For this review, use the dimensioned drawing (mm, ordinates from the lowest corner) and the shaded views. Round coordinates to 2 decimals unless told otherwise and drop trailing zeros. Write each loop counter-clockwise with the first axis right and the second up, starting at its lowest first coordinate (ties: lowest second). Pieces come first, ordered by that corner, then holes. Notation, with made-up numbers: (-28, 20) - (23, 20) arc R6 ccw to (23, 31) - close; hole circle Ø1 at (27, 44.25). An arc over 180 degrees is marked (long way). Write each question's results on one line, items separated by ' | '.
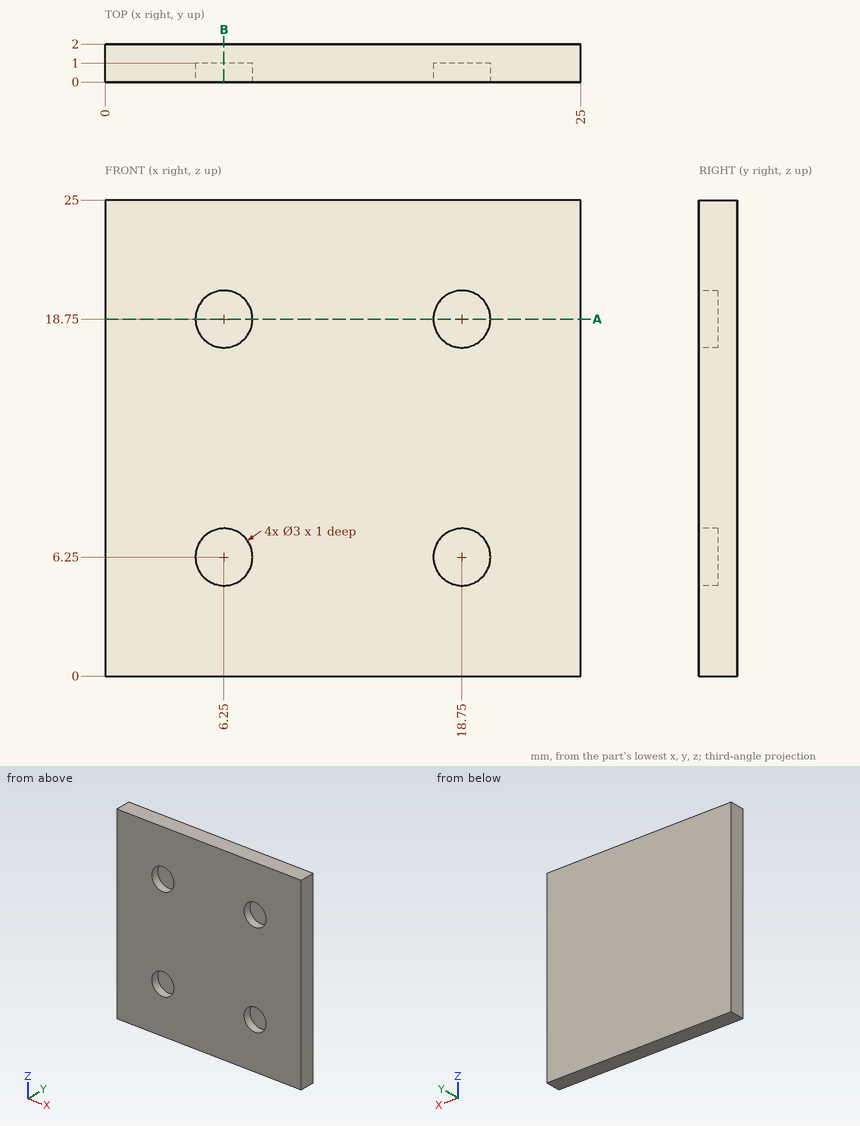
Q1. For probe 1 along Z at (x, y) = (18.75, 0.6); probe 2 along X at (y, z) = (0.75, 7); probe 3 along Z at (x, y) = (7.5, 0.1), list the stretches that pass through material, from the lowest coordinate up.
Evaluation:
probe 1: z = 0 to 4.75, 7.75 to 17.25, 20.25 to 25 | probe 2: x = 0 to 4.95, 7.55 to 17.45, 20.05 to 25 | probe 3: z = 0 to 5.42, 7.08 to 17.92, 19.58 to 25
Q2. We need section A-A (z = 18.75). State the section outline as (x, y) points.
Evaluation:
outline: (0, 0) - (4.75, 0) - (4.75, 1) - (7.75, 1) - (7.75, 0) - (17.25, 0) - (17.25, 1) - (20.25, 1) - (20.25, 0) - (25, 0) - (25, 2) - (0, 2) - close
Q3. We need section B-B (x = 6.25). State the section outline as (y, z) points, plus the area to 3 significant figures.
Evaluation:
outline: (0, 0) - (2, 0) - (2, 25) - (0, 25) - (0, 20.25) - (1, 20.25) - (1, 17.25) - (0, 17.25) - (0, 7.75) - (1, 7.75) - (1, 4.75) - (0, 4.75) - close | area: 44.0 mm^2
Q4. Insertion check: P1, Ø1.8, axis at x = 18.75, z = 18.75, coming from the -Y side. The pin has a flat end and moves straight along its axis. Give the tip position at first contact, or say it passes through.
Evaluation:
P1: stops at y = 1
